Verification items for this drawing (mm, ordinates from the low corner). A direction names the side the tool comes from. Round coordinates to 2 decimals unless told otherwise and drop trailing zeros. Order: outer loops, then holes, each group sorted by start corner. A loop starts at its lowest first (then second) coordinate and runs counter-clockwise, first axis right, second up. Notation, with made-up numbers: (-19, 36.5) - (32, 36.5) arc R32 cw to (32, 69.5) - close; hole circle Ø6 at (43, 57.5). An arc over 180 degrees is marked (long way). Return JSON: item names as keys, results as strings. Group by question number.
Q1. Sectioned sample at A-A, the plane y = 20. Record the cut outline in (x, z), then the cut area to 3 significant figures.
Q2. Sectioned sample at D-D, the plane y = 13. Record the cut outline in (x, z), then the cut area to 3 significant figures.
Q3. Sectioned sample at C-C, the plane x = 100. Record the cut outline in (y, z).
Q4. Gauge pin test, flat ends, axial feed: pin 1 Ø3 at (x, y) = (81, 22) entering from +Z; pin 2 Ø3 at (x, y) = (88, 10.5) entering from -Z; pin 3 Ø6 at (x, z) = (95, 25) entering from -Y; pin 4 Ø8 at (y, z) = (20, 59.5) entering from +X. Record the tip position at first contact, or that the pin passes through.
Q5. Sectioned sample at B-B, the plane z = 100. Record the cut outline in (x, y).
Q6. Material ranges on line 1 along Y through (x, z) = (8, 100); line 2 along Z through (x, y) = (60.5, 16); line 3 along Y through (x, z) = (100, 16.5), recorded low to high.
Q7. Draft check along Z on the marked faces 1, 2, 3 and 4. Enter one of: pulls with the +Z half, pulls with the -Z half, needs draft (parallel to the pull), parting line crosses it, or undercut.
Q8. Tool access check on the marked faces 5, 6 and 7. Record the directions out of +Z, -Z, +X, -X, +Y, -Y that give a thin tool (end or side, any length) a straight path to the whole face; none if there is none.
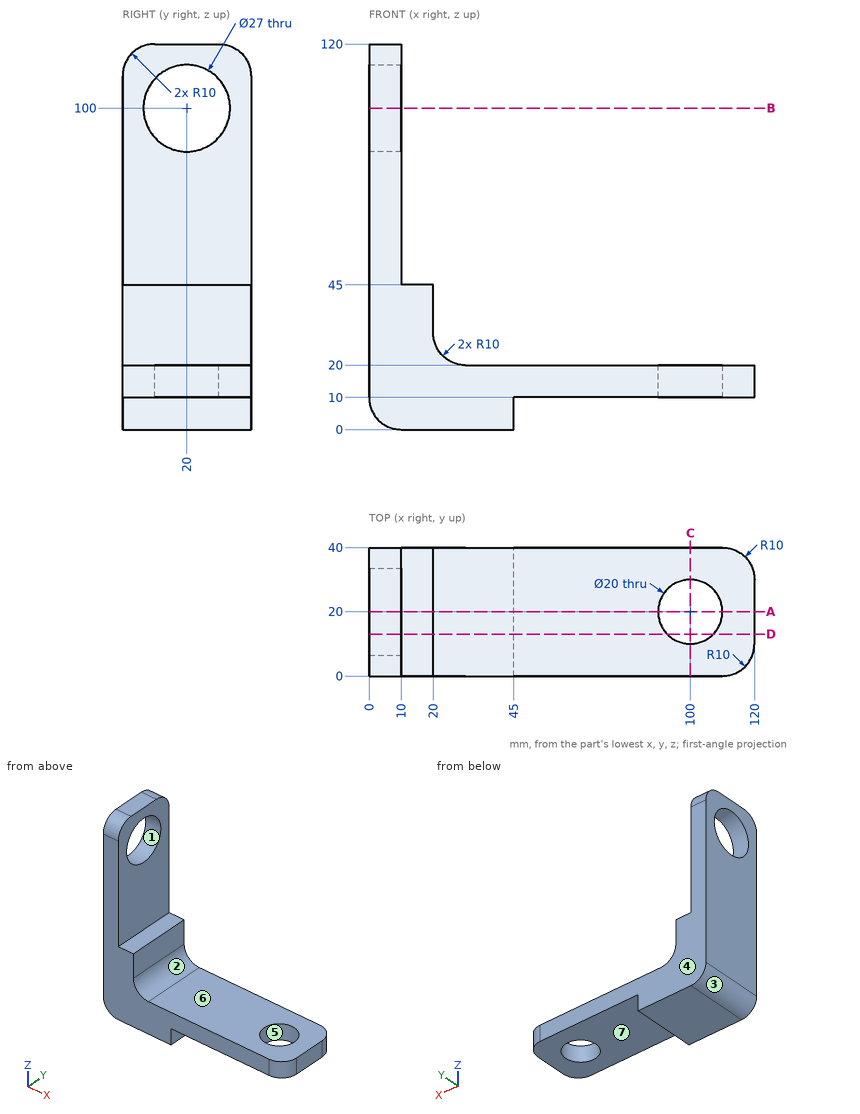
Reply:
{
 "1": {"outline": "(0, 10) arc R10 ccw to (10, 0) - (45, 0) - (45, 10) - (90, 10) - (90, 20) - (30, 20) arc R10 cw to (20, 30) - (20, 45) - (10, 45) - (10, 86.5) - (0, 86.5) - close; (0, 113.5) - (10, 113.5) - (10, 120) - (0, 120) - close; (110, 10) - (120, 10) - (120, 20) - (110, 20) - close", "area": "2,430 mm^2"},
 "2": {"outline": "(0, 10) arc R10 ccw to (10, 0) - (45, 0) - (45, 10) - (92.86, 10) - (92.86, 20) - (30, 20) arc R10 cw to (20, 30) - (20, 45) - (10, 45) - (10, 88.46) - (0, 88.46) - close; (0, 111.54) - (10, 111.54) - (10, 120) - (0, 120) - close; (107.14, 10) - (120, 10) - (120, 20) - (107.14, 20) - close", "area": "2,530 mm^2"},
 "3": {"outline": "(0, 10) - (10, 10) - (10, 20) - (0, 20) - close; (30, 10) - (40, 10) - (40, 20) - (30, 20) - close"},
 "4": {"pin 1": "z = 20", "pin 2": "z = 10", "pin 3": "through", "pin 4": "x = 10"},
 "5": {"outline": "(0, 0) - (10, 0) - (10, 6.5) - (0, 6.5) - close; (0, 33.5) - (10, 33.5) - (10, 40) - (0, 40) - close"},
 "6": {"line 1": "0 to 6.5, 33.5 to 40", "line 2": "10 to 20", "line 3": "0 to 10, 30 to 40"},
 "7": {"face 1": "undercut", "face 2": "pulls with the +Z half", "face 3": "pulls with the -Z half", "face 4": "needs draft"},
 "8": {"face 5": "+Z, -Z", "face 6": "+Z, +X, +Y, -Y", "face 7": "-Z, +X, +Y, -Y"}
}
